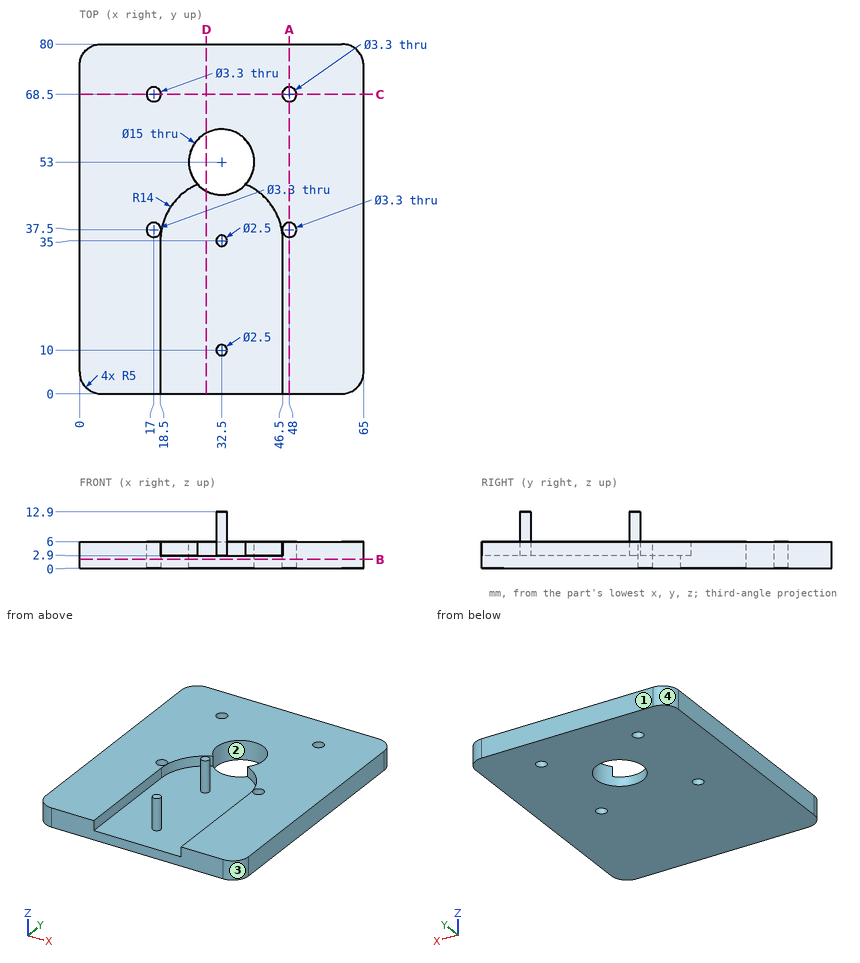
Design review of the part shown in the three views and the two pictorial views. Dimensions are in mm from the part's minimum x, y and z. Round coordinates to 2 decimals unless told otherwise and drop trailing zeros. Write each loop counter-clockwise with the first axis right and the second up, starting at its lowest first coordinate (ties: lowest second). Pieces come first, ordered by that corner, then holes. Notation, with made-up numbers: (42, 89.25) -> (71, 89.25) arc R31 ccw to (71, 124.25) -> close; hole circle Ø6 at (80, 17). An arc over 180 degrees is marked (long way). Write item = value, one per line. Start each with the question number.
1) Mouldability with a two-part tool opening along X and no side actions: class the marked faces 1, 2, 3 and 4 as +X half, -X half, draft (parallel to the pull), parting line (faces both ways), or undercut.
2) Clearance check with flat-ended pins moving along their axes: pin 1 (4 mm diameter, centred on x = 48, y = 37.5, fed in from -Z); pin 2 (1.5 mm diameter, centred on x = 31.5, y = 19.5, fed in from +Z); pin 3 (10 mm diameter, centred on x = 8.5, y = 23, fed in from +Z). State where each tip first meets the part, or that it passes through.
3) Take a section at C-C, the plane y = 68.5. State the section outline as (x, z) points, plus the area to 3 significant figures.
4) Take a section at B-B, the plane z = 2. State the section outline as (x, y) points.
5) Wall thickness on probe 1 along X at (y, z) = (68.5, 1.65); probe 2 along Y at (x, z) = (32.5, 4); probe 3 along Y at (x, z) = (17, 4.5): over which ranges is each line inside the solid? List them lowest first. Write a range as from..to.
6) Take a section at A-A, the plane x = 48. State the section outline as (y, z) points.
7) Take a section at D-D, the plane x = 29. State the section outline as (y, z) points.
Results list:
q1.face_1 = draft
q1.face_2 = undercut
q1.face_3 = +X half
q1.face_4 = -X half
q2.pin_1 = 0
q2.pin_2 = 2.9
q2.pin_3 = 6
q3.outline = (0, 0) -> (15.35, 0) -> (15.35, 6) -> (0, 6) -> close; (18.65, 0) -> (46.35, 0) -> (46.35, 6) -> (18.65, 6) -> close; (49.65, 0) -> (65, 0) -> (65, 6) -> (49.65, 6) -> close
q3.area = 350 mm²
q4.outline = (0, 5) arc R5 ccw to (5, 0) -> (60, 0) arc R5 ccw to (65, 5) -> (65, 75) arc R5 ccw to (60, 80) -> (5, 80) arc R5 ccw to (0, 75) -> close; hole circle Ø3.3 at (17, 37.5); hole circle Ø3.3 at (17, 68.5); hole circle Ø15 at (32.5, 53); hole circle Ø3.3 at (48, 37.5); hole circle Ø3.3 at (48, 68.5)
q5.probe_1 = 0..15.35, 18.65..46.35, 49.65..65
q5.probe_2 = 8.75..11.25, 33.75..36.25, 60.5..80
q5.probe_3 = 0..35.85, 39.15..66.85, 70.15..80
q6.outline = (0, 0) -> (35.85, 0) -> (35.85, 6) -> (0, 6) -> close; (39.15, 0) -> (66.85, 0) -> (66.85, 6) -> (39.15, 6) -> close; (70.15, 0) -> (80, 0) -> (80, 6) -> (70.15, 6) -> close
q7.outline = (0, 0) -> (46.37, 0) -> (46.37, 2.9) -> (0, 2.9) -> close; (59.63, 0) -> (80, 0) -> (80, 6) -> (59.63, 6) -> close
